from build123d import *

# Parameters (mm, degrees)
F0_R     = 10.7864986288
F1_DEPTH = 4.318
F2_R     = 6.2270192231
F3_DEPTH = 3.048
F4_R     = 10.6768853932
F4_R_2   = 6.2270192231
F5_DEPTH = 4.826


with BuildPart() as f1:
    # F0 (on Right) → F1 (new body)
    with BuildSketch(Plane.YZ):
        Circle(F0_R)
    extrude(amount=F1_DEPTH)

    # F2 (on face) → F3 (join)
    with BuildSketch(Plane(origin=(0, 0, 0), x_dir=(0, -1, 0), z_dir=(-1, 0, 0))):
        Circle(F2_R)
    extrude(amount=F3_DEPTH)

    # F4 (on face) → F5 (join)
    with BuildSketch(Plane(origin=(-3.048, 0, 0), x_dir=(0, -1, 0), z_dir=(-1, 0, 0))):
        Circle(F4_R)
        Circle(F4_R_2, mode=Mode.SUBTRACT)
        Circle(F4_R_2)
    extrude(amount=F5_DEPTH)


solid = f1.part
Could you check a few things on this model? Use its own coordinates, in mm. A direction names the side the tool comes from. Round coordinates to 2 decimals unless told otherwise and drop trailing zeros. Write each loop counter-clockwise with the first axis right and the second up, starting at its lowest first coordinate (ties: lowest second). Pieces come first, ordered by that corner, then holes. Notation, with made-up numbers: (85.5, 11) - (126.5, 11) arc R10 ccw to (126.5, 16) - close; hole circle Ø4 at (8.25, 16). An arc over 180 degrees is marked (long way). Put each result on its own line as item: value. Start each with the question number.
(1) I need wall thicknesses on probe 1 along X at (y, z) = (6.75, 3.5); probe 2 along Z at (x, y) = (1, 0); probe 3 along Y at (x, z) = (0.25, -3.5). Which ranges of each line are inside material? Lowest first, please.
(2) For faces 4 (the cylindrical face through (2.129, 5.799, 9.095)), 5 (the cylindrical face through (-5.43, -4.93, -9.47)), 6 (the cylindrical face through (-1.503, 0.811, 6.174)), which set-ups out of +Z, -Z, +X, -X, +Y, -Y let a thin tool reach every point of the face, with its end or its side?
(3) I want a section at C-C, the plane z = -7. Please give me the cut outline in (x, y), plus the area to 3 significant figures.
(4) I want a section at A-A, the plane y = 0. Please give me the cut outline in (x, z).
(5) Will these pins go through, and if not, where does the flat tip stop? pin 1 (1 mm diameter, centred on x = -3, z = 2, fed in from +Y); pin 2 (3 mm diameter, centred on x = 0.5, y = -5.5, fed in from -Z); pin 3 (5 mm diameter, centred on x = -0.5, z = 6, fed in from +Y).
(6) I want a section at D-D, the plane x = -4.75. Please give me the cut outline in (y, z).
(7) Thinking about a two-plate mould opening in X: for faces 1 (the flat face through (0, 5, -5)), 2 (the flat face through (4.318, 0, 0)), 3 (the flat face through (-7.874, 0, 0)), which applies, released by +X, released by -X, zero draft, split by the parting line, or undercut?
Here are the results:
1. probe 1: x = -7.87 to -3.05, 0 to 4.32
1. probe 2: z = -10.79 to 10.79
1. probe 3: y = -10.2 to 10.2
2. face 4: +X, -X
2. face 5: -X
2. face 6: none
3. outline: (-7.87, -8.06) - (-3.05, -8.06) - (-3.05, 8.06) - (-7.87, 8.06) - close; (0, -8.21) - (4.32, -8.21) - (4.32, 8.21) - (0, 8.21) - close
3. area: 149 mm^2
4. outline: (-7.87, -10.68) - (-3.05, -10.68) - (-3.05, -6.23) - (0, -6.23) - (0, -10.79) - (4.32, -10.79) - (4.32, 10.79) - (0, 10.79) - (0, 6.23) - (-3.05, 6.23) - (-3.05, 10.68) - (-7.87, 10.68) - close
5. pin 1: stops at y = 10.57
5. pin 2: stops at z = -10.02
5. pin 3: stops at y = 10.19
6. outline: circle Ø21.35 at (0, 0)
7. face 1: undercut
7. face 2: released by +X
7. face 3: released by -X
